Could you check a few things on this model? Use its own coordinates, in mm. Face numbers are marked on the shaded views. A direction names the side the tool comes from. Round coordinates to 2 decimals unless told otherwise and drop trailing zeros. Order: outer loops, then holes, each group sorted by start corner. A loop starts at its lowest first (then second) coordinate and runs counter-clockwise, first axis right, second up. Notation, with made-up numbers: (54.25, 62) - (64.25, 62) arc R19 cw to (64.25, 70) - close; hole circle Ø1 at (-33, 47.25). An arc over 180 degrees is marked (long way). Return JSON: item names as keys, results as strings. Group by question number.
from build123d import *

# Parameters (mm, degrees)
CROQUIS1_R              = 6
CROQUIS1_R_2            = 4.5
SALIENTE_EXTRUIR1_DEPTH = 25
CROQUIS2_R              = 6
CROQUIS2_R_2            = 4
SALIENTE_EXTRUIR2_DEPTH = 25
CROQUIS3_R              = 4.5
CORTAR_EXTRUIR1_DEPTH   = 51.0000001


with BuildPart() as part:
    # Croquis1 → Saliente-Extruir1 (new body, symmetric)
    with BuildSketch(Plane.XY):
        Circle(CROQUIS1_R)
        Circle(CROQUIS1_R_2, mode=Mode.SUBTRACT)
    extrude(amount=SALIENTE_EXTRUIR1_DEPTH, both=True)

    # Croquis2 → Saliente-Extruir2 (add)
    with BuildSketch(Plane(origin=(0, 0, 0), x_dir=(1, 0, 0), z_dir=(0, 1, 0))):
        Circle(CROQUIS2_R)
        Circle(CROQUIS2_R_2, mode=Mode.SUBTRACT)
    extrude(amount=SALIENTE_EXTRUIR2_DEPTH)

    # Croquis3 → Cortar-Extruir1 (cut, through all)
    with BuildSketch(Plane.XY.offset(25)):
        Circle(CROQUIS3_R)
    extrude(amount=-CORTAR_EXTRUIR1_DEPTH, mode=Mode.SUBTRACT)


solid = part.part
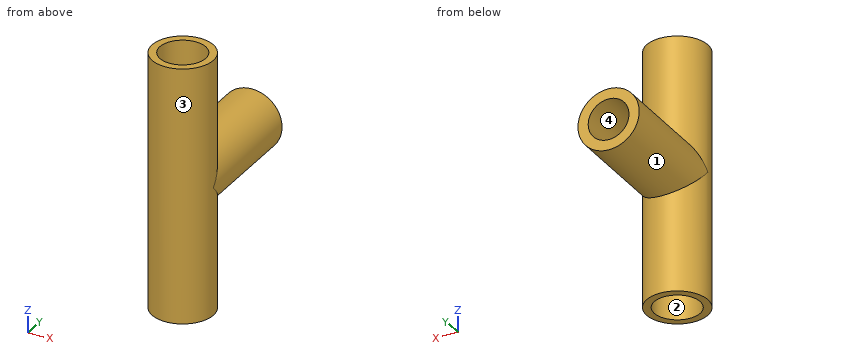
1) I want a section at D-D, the plane y = 16.5. List the corners of the cut face in (x, z) for me, plus the area to 3 significant figures.
2) Will these pins go through, and if not, where does the flat tip stop? pin 1 (2 mm diameter, centred on y = -1.5, z = -18, fed in from +X); pin 2 (1.5 mm diameter, centred on y = 17, z = 1.5, fed in from -X); pin 3 (6 mm diameter, centred on x = 4.5, z = 13.5, fed in from -Y).
3) For the marked faces 1 and 2, which set-ups out of +Z, -Z, +X, -X, +Y, -Y let a thin tool reach every point of the face, with its end or its side?
4) If I drill on line 1 along Z through (x, y) = (0, 20); line 2 along Y through (x, z) = (2, 13.5); line 3 along Z through (x, y) = (-3, 18), over which ranges is the centre line in solid material (lowest first)? Write a range as from..to.
5) I want a section at C-C, the plane z = 0. List the corners of the cut face in (x, y) for me, plus the area to 3 significant figures.
6) I want a section at B-B, the plane y = 3.5. List the corners of the cut face in (x, z) for me, plus the area to 3 significant figures.
7) We'd pull the mould along X, two halves only. Please class the marked faces 3 and 4: +X half, -X half, draft (parallel to the pull), parting line (faces both ways), or undercut.
8) I want a section at A-A, the plane x = 0. List the corners of the cut face in (y, z) for me.
Outcome:
{
 "1": {"outline": "circle Ø12 at (0, 0); hole circle Ø8 at (0, 0)", "area": "62.8 mm^2"},
 "2": {"pin 1": "x = 5.98", "pin 2": "x = -5.95", "pin 3": "y = -5.81"},
 "3": {"face 1": "+Y", "face 2": "+Z, -Z"},
 "4": {"line 1": "-6..-4, 4..6", "line 2": "-5.66..-4.03, 4.03..5.66", "line 3": "-5.2..-2.65, 2.65..5.2"},
 "5": {"outline": "(-6, 0) arc R6 ccw to (6, 0) - (6, 25) - (4, 25) - (4, 4.47) arc R6 ccw to (-4, 4.47) - (-4, 25) - (-6, 25) - close; hole circle Ø9 at (0, 0)", "area": "137 mm^2"},
 "6": {"outline": "(-4.87, -25) - (-2.83, -25) - (-2.83, 25) - (-4.87, 25) - (-4.87, 3.5) arc R6 ccw to (-4.87, -3.5) - close; (2.83, -25) - (4.87, -25) - (4.87, -3.5) arc R6 ccw to (4.87, 3.5) - (4.87, 25) - (2.83, 25) - close", "area": "215 mm^2"},
 "7": {"face 3": "parting line", "face 4": "undercut"},
 "8": {"outline": "(-6, -25) - (-4.5, -25) - (-4.5, 25) - (-6, 25) - close; (4.5, -25) - (6, -25) - (6, -6) - (25, -6) - (25, -4) - (6, -4) - (6, 4) - (25, 4) - (25, 6) - (6, 6) - (6, 25) - (4.5, 25) - close"}
}
